Verification items for the finished model (mm, model axes). A direction names the side the tool comes from. Round coordinates to 2 decimals unless told otherwise and drop trailing zeros. Order: outer loops, then holes, each group sorted by start corner. A loop starts at its lowest first (then second) coordinate and runs counter-clockwise, first axis right, second up. Notation, with made-up numbers: (7, 78) -> (62, 78) arc R24 cw to (62, 112) -> close; hole circle Ø7 at (55, 82.5). An arc over 180 degrees is marked (long way). Answer in a Markdown table with one row per item. Add a question column.
Autodesk Inventor part; units mm, degrees
ref_plane "Work Plane1" through (0, 0, -30) normal (0, 0, 1) x (1, 0, 0)
ref_plane "YZ Plane" through (0, 0, 0) normal (1, 0, 0) x (0, 1, 0)
ref_plane "XZ Plane" through (0, 0, 0) normal (0, 1, 0) x (-1, 0, 0)
sketch "Sketch2" plane through (0, 0, 0) normal (0, 0, 1) x (1, 0, 0)
  line L0 (0, 0) -> (25, 0) construction
  circle A0 centre (0, 0) radius 7.5 construction
  line L1 (15.1273, 0) -> (20.0637, 8.55) construction
  line L2 (20.0637, 8.55) -> (29.9363, 8.55) construction
  line L3 (29.9363, 8.55) -> (34.8727, 0) construction
  line L4 (34.8727, 0) -> (29.9363, -8.55) construction
  line L5 (29.9363, -8.55) -> (20.0637, -8.55) construction
  line L6 (20.0637, -8.55) -> (15.1273, 0) construction
  line L7 (0, 0) -> (0, 26) construction
  line L8 (0, 26) -> (25, 26) construction
  line L9 (-7.3485, 1.5) -> (-13.3485, 1.5)
  line L10 (-13.3485, 1.5) -> (-13.3485, -1.5) construction
  line L11 (-13.3485, -1.5) -> (-7.3485, -1.5)
  line L12 (-13.3485, -1.5) -> (-13.3485, -4)
  line L13 (-13.3485, 1.5) -> (-13.3485, 4)
  line L14 (-5, 23) -> (-5, 8.6603)
  arc A1 (-5, 8.6603) -> (-9.1652, 4) centre (0, 0) ccw
  line L15 (-13.3485, 4) -> (-9.1652, 4)
  line L16 (-13.3485, -4) -> (-9.1652, -4)
  arc A2 (-9.1652, 4) -> (-9.1652, -4) centre (0, 0) ccw construction
  arc A3 (-9.1652, -4) -> (7.1414, 7) centre (0, 0) ccw
  line L17 (-5, 23) -> (40, 23)
  arc A4 (-7.3485, -1.5) -> (-7.3485, 1.5) centre (0, 0) ccw
  circle A5 centre (25, 0) radius 5 construction
  circle A6 centre (25, 0) radius 6 construction
  line L18 (40, 23) -> (40, 7)
  line L19 (40, 7) -> (7.1414, 7)
  line L20 (40, 15) -> (-5, 15) construction
  line L21 (40, 19) -> (-5, 19) construction
  line L22 (-5, 11) -> (40, 11) construction
  dimension "d32" = 25
  dimension "d33" = 15
  dimension "d34" = 17.1
  dimension "d35" = 26
  dimension "d36" = 6
  dimension "d37" = 2.5
  dimension "d38" = 3
  dimension "d39" = 2.5
  dimension "d40" = 3
  dimension "d41" = 10
  dimension "d42" = 1
  dimension "d43" = 16
  dimension "d44" = 8
  dimension "d45" = 5
  dimension "d46" = 45
extrude "Extrusion6" add sketch "Sketch2" against normal blind 60
fillet "Fillet1" radius 2 2 edges at (7.1414, 7, -30) (-5, 8.6603, -30)
ref_plane "Work Plane1" through (0, 0, -30) normal (0, 0, 1) x (1, 0, 0)
sketch "Sketch4" plane through (40, 7, 0) normal (1, 0, 0) x (0, 0, -1)
  line L0 (0, 16) -> (0, 0)
  line L1 (60, 16) -> (60, 0)
  line L2 (0, 8) -> (60, 8) construction
  circle A0 centre (8.5, 8) radius 4
  line L3 (4.5, 4) -> (8.5, 4)
  line L4 (8.5, 4) -> (8.5, 12)
  line L5 (8.5, 12) -> (4.5, 12)
  line L6 (4.5, 12) -> (4.5, 4)
  line L7 (4.5, 4) -> (8.5, 12) construction
  line L8 (8.5, 4) -> (4.5, 12) construction
  line L9 (3.3, 4) -> (2.4, 4)
  line L10 (2.4, 4) -> (2.4, 12)
  line L11 (2.4, 12) -> (3.3, 12)
  line L12 (3.3, 12) -> (3.3, 4)
  line L13 (3.3, 4) -> (2.4, 12) construction
  line L14 (2.4, 4) -> (3.3, 12) construction
  circle A1 centre (53.5, 8) radius 4
  line L15 (49.5, 4) -> (53.5, 4)
  line L16 (53.5, 4) -> (53.5, 12)
  line L17 (53.5, 12) -> (49.5, 12)
  line L18 (49.5, 12) -> (49.5, 4)
  line L19 (49.5, 4) -> (53.5, 12) construction
  line L20 (53.5, 4) -> (49.5, 12) construction
  line L21 (48.3, 4) -> (47.4, 4)
  line L22 (47.4, 4) -> (47.4, 12)
  line L23 (47.4, 12) -> (48.3, 12)
  line L24 (48.3, 12) -> (48.3, 4)
  line L25 (48.3, 4) -> (47.4, 12) construction
  line L26 (47.4, 4) -> (48.3, 12) construction
  line L27 (43.4, 3) -> (16.6, 3)
  line L28 (16.6, 3) -> (16.6, 13)
  line L29 (16.6, 13) -> (43.4, 13)
  line L30 (43.4, 13) -> (43.4, 3)
  line L31 (43.4, 3) -> (16.6, 13) construction
  line L32 (16.6, 3) -> (43.4, 13) construction
  line L33 (47.4, 8) -> (43.4, 8) construction
  line L34 (12.5, 8) -> (16.6, 8) construction
  point P0 (0, -7)
  point P1 (6.5, 8)
  point P2 (2.85, 8)
  point P3 (51.5, 8)
  point P4 (47.85, 8)
  point P5 (30, 8)
  dimension "d52" = 8
  dimension "d53" = 0.9
  dimension "d54" = 1.2
  dimension "d55" = 2.4
  dimension "d58" = 45
  dimension "d63" = 10
  dimension "d65" = 4
extrude "Extrusion7" cut sketch "Sketch4" against normal up to next
properties part number "X_base"
1) Cross-section at C-C, the plane x = 13. Record the boundary of the cut face in (y, z).
2) Depth check by flat-ended pin: P1, Ø8, axis at y = -6.5, z = -7, coming from the -X side; P2, Ø2, axis at x = -11.5, z = -42, coming from the +Y side; P3, Ø2, axis at x = 2, z = -21.5, coming from the -Y side; P4, Ø3, axis at x = 21, z = -6, coming from the -Y side. Enter the tip coordinate at first touch or a pass-through.
3) Tool access check on faces 3 (the face through (18, 19, -7)), 4 (the face through (-10, 1.5, -30)), 5 (the face through (-11, -4, -30)), 6 (the face through (-11, 4, -30)). Record the directions out of +Z, -Z, +X, -X, +Y, -Y that give a thin tool (end or side, any length) a straight path to the whole face; none if there is none.
4) Draft check along Z on faces 1 (the face through (-8, 6, -30)), 2 (the face through (18, 15, -48.3)). Enter one of: +Z half, -Z half, draft (parallel to the pull), parting line (faces both ways), or undercut.
5) Cross-section at A-A, the plane x = 0. Record the boundary of the cut face in (y, z), and give its area (3 significant figures).
6) Thickness scan on L1, parallel to Y at x = 0, z = -33; L2, parallel to Z at x = 13.5, y = 12; L3, parallel to Y at x = 25, z = -20.5. Record the ranges inside material, lowest first. Write a range as [from, to].
7) Cross-section at B-B, the plane y = 15. Record the boundary of the cut face in (x, z), and give its area (3 significant figures).
8) Cross-section at D-D, the plane z = -10. Record the boundary of the cut face in (x, y).
Results below:
| question | item | result |
|---|---|---|
| 1 | outline | (7, -60) -> (23, -60) -> (23, 0) -> (7, 0) -> close; hole (10, -43.4) -> (20, -43.4) -> (20, -16.6) -> (10, -16.6) -> close; hole (11, -53.5) arc R4 ccw to (19, -53.5) -> (19, -49.5) -> (11, -49.5) -> close; hole (11, -48.3) -> (19, -48.3) -> (19, -47.4) -> (11, -47.4) -> close; hole (11, -8.5) arc R4 ccw to (19, -8.5) -> (19, -4.5) -> (11, -4.5) -> close; hole (11, -3.3) -> (19, -3.3) -> (19, -2.4) -> (11, -2.4) -> close |
| 2 | P1 | x = -13.35 |
| 2 | P2 | y = 4 |
| 2 | P3 | y = -9.95 |
| 2 | P4 | y = 7 |
| 3 | face 3 | +X, -X |
| 3 | face 4 | +Z, -Z, -X |
| 3 | face 5 | +Z, -Z, -X, -Y |
| 3 | face 6 | +Z, -Z, -X, +Y |
| 4 | face 1 | draft |
| 4 | face 2 | undercut |
| 5 | outline | (-10, -60) -> (-7.5, -60) -> (-7.5, 0) -> (-10, 0) -> close; (7.5, -60) -> (23, -60) -> (23, 0) -> (7.5, 0) -> close; hole (10, -43.4) -> (20, -43.4) -> (20, -16.6) -> (10, -16.6) -> close; hole (11, -53.5) arc R4 ccw to (19, -53.5) -> (19, -49.5) -> (11, -49.5) -> close; hole (11, -48.3) -> (19, -48.3) -> (19, -47.4) -> (11, -47.4) -> close; hole (11, -8.5) arc R4 ccw to (19, -8.5) -> (19, -4.5) -> (11, -4.5) -> close; hole (11, -3.3) -> (19, -3.3) -> (19, -2.4) -> (11, -2.4) -> close |
| 5 | area | 683 mm² |
| 6 | L1 | [-10, -7.5], [7.5, 10], [20, 23] |
| 6 | L2 | [-60, -56.15], [-49.5, -48.3], [-47.4, -43.4], [-16.6, -11.15], [-4.5, -3.3], [-2.4, 0] |
| 6 | L3 | [7, 10], [20, 23] |
| 7 | outline | (-5, -60) -> (40, -60) -> (40, -57.5) -> (-5, -57.5) -> close; (-5, -49.5) -> (40, -49.5) -> (40, -48.3) -> (-5, -48.3) -> close; (-5, -47.4) -> (40, -47.4) -> (40, -43.4) -> (-5, -43.4) -> close; (-5, -16.6) -> (40, -16.6) -> (40, -12.5) -> (-5, -12.5) -> close; (-5, -4.5) -> (40, -4.5) -> (40, -3.3) -> (-5, -3.3) -> close; (-5, -2.4) -> (40, -2.4) -> (40, 0) -> (-5, 0) -> close |
| 7 | area | 693 mm² |
| 8 | outline | (-13.35, -4) -> (-9.17, -4) arc R10 ccw (long way) to (9.09, 4.17) arc R2 cw to (10.91, 7) -> (40, 7) -> (40, 11.29) -> (-5, 11.29) -> (-5, 9.75) arc R2 cw to (-5.83, 8.12) arc R10 ccw to (-9.17, 4) -> (-13.35, 4) -> (-13.35, 1.5) -> (-7.35, 1.5) arc R7.5 cw (long way) to (-7.35, -1.5) -> (-13.35, -1.5) -> close; (-5, 18.71) -> (40, 18.71) -> (40, 23) -> (-5, 23) -> close |
